Here's how the part is built. I have some questions about the finished solid (model axes, mm). Round coordinates to 2 decimals unless told otherwise and drop trailing zeros. Write each loop counter-clockwise with the first axis right and the second up, starting at its lowest first coordinate (ties: lowest second). Pieces come first, ordered by that corner, then holes. Notation, with made-up numbers: (77.25, 29) -> (113.25, 29) arc R14 ccw to (113.25, 55) -> close; hole circle Ø5 at (-36.5, -2). An arc over 180 degrees is marked (long way). Answer as CSV lines item,"result".
Autodesk Inventor part; units mm, degrees
ref_plane "YZ Plane" through (0, 0, 0) normal (1, 0, 0) x (0, 1, 0)
sketch "Эскиз1" plane through (0, 0, 0) normal (1, 0, 0) x (0, 1, 0)
  line L0 (95, -77) -> (95, 77)
  line L1 (82, 90) -> (-82, 90)
  line L2 (-95, 77) -> (-95, -77)
  line L3 (-82, -90) -> (82, -90)
  arc A0 (82, -90) -> (95, -77) centre (82, -77) ccw
  arc A1 (-95, -77) -> (-82, -90) centre (-82, -77) ccw
  arc A2 (-82, 90) -> (-95, 77) centre (-82, 77) ccw
  arc A3 (95, 77) -> (82, 90) centre (82, 77) ccw
  line L4 (-82, 90) -> (82, 90)
  line L5 (82, 68) -> (-82, 68)
  line L6 (-82, 68) -> (-82, 86)
  line L7 (-82, 86) -> (82, 86)
  line L8 (-82, -90) -> (82, -90)
  line L9 (82, -86) -> (82, -68)
  line L10 (82, -68) -> (-82, -68)
  line L11 (-82, -68) -> (-82, -86)
  line L12 (-82, -86) -> (82, -86)
  line L13 (82, 86) -> (82, 68)
  line L14 (82, 68) -> (72, 68)
  line L15 (72, 86) -> (82, 86)
  line L16 (-82, 68) -> (-72, 68)
  line L17 (-72, 68) -> (-72, 86)
  line L18 (-72, 86) -> (-82, 86)
  line L19 (-82, 86) -> (-82, 68)
  line L20 (-72, 86) -> (-68.8341, 86)
  line L21 (-68.8341, 86) -> (-68.8341, 84.5)
  line L22 (-68.8341, 84.5) -> (-72, 84.5)
  line L23 (-72, 84.5) -> (-72, 86)
  line L24 (-72, 84.5) -> (-12, 84.5)
  line L25 (-12, 84.5) -> (-12, 69.5)
  line L26 (-12, 69.5) -> (-72, 69.5)
  line L27 (-72, 69.5) -> (-72, 84.5)
  line L28 (82, 86) -> (72, 86)
  line L29 (72, 86) -> (72, 68)
  line L30 (72, 68) -> (82, 68)
  line L31 (82, 68) -> (82, 86)
  line L32 (72, 84.5) -> (12, 84.5)
  line L33 (12, 84.5) -> (12, 69.5)
  line L34 (12, 69.5) -> (72, 69.5)
  line L35 (72, 69.5) -> (72, 84.5)
  line L36 (-42, 68) -> (-54.5, 68)
  line L37 (-54.5, 8) -> (-29.5, 8)
  line L38 (-29.5, 8) -> (-29.5, 68)
  line L39 (-29.5, 68) -> (-54.5, 68)
  line L40 (-54.5, 68) -> (-54.5, 8)
  point P0 (0, 0)
  point P1 (-95, 90)
  point P2 (95, 90)
  point P3 (-95, -90)
  dimension "d6" = 180
  dimension "d7" = 190
  dimension "d8" = 13
  dimension "d9" = 13
  dimension "d11" = 18
  dimension "d19" = 10
  dimension "d20" = 1.5
  dimension "d21" = 60
  dimension "d22" = 15
  dimension "d23" = 10
  dimension "d24" = 60
  dimension "d26" = 60
  dimension "d27" = 25
extrude "Выдавливание1" add sketch "Эскиз1" along normal blind 3 contours A0 L3 A1 L2 A2 L1 A3 L0 | L38 L37 L40 L5
properties part number "основа_прототип"
Item 1: Suppose I cut it at A-A, the plane x = 1.95. List the corners of the cut face in (y, z) for me, then the cut area to 3 significant figures.
Results found:
outline,"(-95, -77) arc R13 ccw to (-82, -90) -> (82, -90) arc R13 ccw to (95, -77) -> (95, 77) arc R13 ccw to (82, 90) -> (-82, 90) arc R13 ccw to (-95, 77) -> close; hole (-82, -86) -> (82, -86) -> (82, -68) -> (-82, -68) -> close; hole (-82, 68) -> (82, 68) -> (82, 86) -> (-82, 86) -> close"
area,"28,200 mm²"
Item 2: Suppose I cut it at B-B, the plane y = -57.5. List the corners of the cut face in (x, z) for me.
Results found:
outline,"(0, -90) -> (3, -90) -> (3, -86) -> (0, -86) -> close; (0, -68) -> (3, -68) -> (3, 68) -> (0, 68) -> close; (0, 86) -> (3, 86) -> (3, 90) -> (0, 90) -> close"
Item 3: Will this pin go through, and if not, where does the flat tip stop? pin 1 (1.5 mm diameter, centred on x = 1.5, z = 81, fed in from +Y).
Results found:
pin 1,"stops at y = 94.59"
Item 4: I need wall thicknesses on L1, parallel to Z at x = 1.6, y = 20; L2, parallel to Y at x = 2.6, z = 68.5. Which ranges of each line are inside material? Lowest first, please.
Results found:
L1,"z = -90 to -86, -68 to 68, 86 to 90"
L2,"y = -95 to -82, 82 to 95"
